The model under review builds one solid part; all positions refer to its coordinate system, in mm. A direction names the side the tool comes from. Coordinates: 2 decimals unless noted, no trailing zeros. Loops run counter-clockwise (first coordinate to the right, second up) from the corner with the lowest first, then second, coordinate; pieces in that order, holes last. Notation, with made-up numbers: (12, 23.25) - (32, 23.25) arc R20 ccw to (32, 48.25) - close; hole circle Ø6 at (82.25, -24.75). An arc over 180 degrees is marked (long way). Answer in a Markdown table with one row per item. Add a question column.
(1) For line 1 along X through (y, z) = (2, 4.25); line 2 along X through (y, z) = (-1.25, 6.5); line 3 along Y through (x, z) = (8.5, 2), list the stretches that pass through material, from the lowest coordinate up.
(2) Machinability: for faces 1 (the flat face through (-15, 7, 4)), 2 (the flat face through (11, -3, 4)), 3 (the flat face through (-23, 2, 4)), 4 (the flat face through (-6, 0, 3)), 5 (the flat face through (-23, -2, 4)), which of the approach directions +Z, -Z, +X, -X, +Y, -Y give a long, thin tool a straight path to every point of the face, cutting with its end or side? Answer none if there is none.
(3) Mouldability with a two-part tool opening along Y and no side actions: class faces 6 (the flat face through (-4, -2.75, 3)), 7 (the flat face through (15, 7, 4)), 8 (the flat face through (-19, 3, 4)) as +Y half, -Y half, draft (parallel to the pull), parting line (faces both ways), or undercut.
(4) For P1, Ø4, axis at x = -34, z = 4.5, coming from the -Y side; P2, Ø2, axis at y = -2.5, z = 5, coming from the +X side; P3, Ø1.5, axis at y = 1.5, z = 5.5, coming from the +X side; P4, Ø3, axis at x = -29.5, z = 5, coming from the +Y side, all flat-tipped, find the tip position at first contact; note any pin that passes through.
(5) We need section C-C on y = -4. Write out the cut boundary in (x, z).
(6) We need section D-D on x = -25.5. Write out the cut boundary in (y, z).
(7) We need section A-A on z = 3. Write out the cut boundary in (x, y).
(8) We need section B-B on x = -5.5. Write out the cut boundary in (y, z), plus the area to 3 significant figures.
from build123d import *

# Parameters (mm, degrees)
F0_W     = 5
F0_H     = 5.5
F1_DEPTH = 7.6
F2_W     = 5
F2_H     = 5.5
F3_DEPTH = 1


with BuildPart() as f1:
    # F0 (on Top) → F1 (new body)
    with BuildSketch(Plane.XY):
        Polygon((-23, -3), (-15, -3), (-15, 3), (-23, 3), (-23, 1.75), (-27.7, 1.75), (-27.7, 2.5), (-31.7, 2.5), (-31.7, 1.75), (-36.4, 1.75), (-36.4, -1.75), (-31.7, -1.75), (-31.7, -2.5), (-27.7, -2.5), (-27.7, -1.75), (-23, -1.75), align=None)
        Polygon((-15, -3), (-15, -10.9), (15, -10.9), (15, -3), (7.3, -3), (7.3, 3), (15, 3), (15, 10.9), (-15, 10.9), (-15, 3), align=None)
        with Locations((-3.5, 0)):
            Rectangle(F0_W, F0_H, mode=Mode.SUBTRACT)
    extrude(amount=F1_DEPTH)

    # F2 (on face) → F3 (join)
    with BuildSketch(Plane.XY.offset(7.6)):
        with Locations((-3.5, 0)):
            Rectangle(F2_W, F2_H)
    extrude(amount=-F3_DEPTH)


solid = f1.part
Outcome:
| question | item | result |
|---|---|---|
| 1 | line 1 | -31.7 to -27.7, -23 to -6, -1 to 7.3 |
| 1 | line 2 | -36.4 to -6, -1 to 7.3 |
| 1 | line 3 | -10.9 to -3, 3 to 10.9 |
| 2 | face 1 | +Z, -Z, -X, +Y |
| 2 | face 2 | +Z, -Z, +X |
| 2 | face 3 | +Z, -Z, +Y |
| 2 | face 4 | -Z |
| 2 | face 5 | +Z, -Z, -Y |
| 3 | face 6 | undercut |
| 3 | face 7 | draft |
| 3 | face 8 | +Y half |
| 4 | P1 | y = -1.75 |
| 4 | P2 | x = 15 |
| 4 | P3 | x = 7.3 |
| 4 | P4 | y = 2.5 |
| 5 | outline | (-15, 0) - (15, 0) - (15, 7.6) - (-15, 7.6) - close |
| 6 | outline | (-1.75, 0) - (1.75, 0) - (1.75, 7.6) - (-1.75, 7.6) - close |
| 7 | outline | (-36.4, -1.75) - (-31.7, -1.75) - (-31.7, -2.5) - (-27.7, -2.5) - (-27.7, -1.75) - (-23, -1.75) - (-23, -3) - (-15, -3) - (-15, -10.9) - (15, -10.9) - (15, -3) - (7.3, -3) - (7.3, 3) - (15, 3) - (15, 10.9) - (-15, 10.9) - (-15, 3) - (-23, 3) - (-23, 1.75) - (-27.7, 1.75) - (-27.7, 2.5) - (-31.7, 2.5) - (-31.7, 1.75) - (-36.4, 1.75) - close; hole (-6, -2.75) - (-1, -2.75) - (-1, 2.75) - (-6, 2.75) - close |
| 8 | outline | (-10.9, 0) - (-2.75, 0) - (-2.75, 6.6) - (2.75, 6.6) - (2.75, 0) - (10.9, 0) - (10.9, 7.6) - (-10.9, 7.6) - close |
| 8 | area | 129 mm² |
